Verification items for the finished model (mm, model axes). Face numbers are marked on the shaded views. Give positions to 0.01 mm unless a question says otherwise; leave off trailing zeros. Write each loop counter-clockwise with the first axis right and the second up, starting at its lowest first coordinate (ties: lowest second). Pieces come first, ordered by that corner, then holes. Notation, with made-up numbers: (-2.5, 57.25) -> (36.5, 57.25) arc R21 cw to (36.5, 74.25) -> close; hole circle Ø4 at (-23, 74). An arc over 180 degrees is marked (long way). Use one line per item in the form item = value. Start each with the question number.
(1) Scan lines: L1, parallel to Y at x = 0, z = 2; L2, parallel to X at y = -16, z = 2; L3, parallel to X at y = -8.5, z = 5.25. Record each from-to range of solid material in increasing order.
(2) Section check A-A, the plane z = 3. Record the cut outline in (x, y), plus the area to 3 significant figures.
(3) Section check B-B, the plane x = 8.5. Record the cut outline in (y, z), plus the area to 3 significant figures.
(4) Release check for a two-part mould opening along X. For the marked faces 1 and 2 record: pulls with the +X half, pulls with the -X half, needs draft (parallel to the pull), parting line crosses it, or undercut.
(5) Depth check by flat-ended pin: pin 1 Ø1 at (y, z) = (2.5, 4) entering from -X; pin 2 Ø8 at (x, y) = (24, 3) entering from +Z; pin 3 Ø20 at (x, y) = (0, 28.87) entering from +Z; pin 4 Ø1.5 at (x, z) = (-17.5, 5.5) entering from -Y. Enter the tip coordinate at first touch or a pass-through.
(6) Section check C-C, the plane y = 37.5. Record the cut outline in (x, z).
(7) Section check D-D, the plane x = -7. Record the cut outline in (y, z), plus the area to 3 significant figures.
from build123d import *

# Parameters (mm, degrees)
F0_R        = 11
F1_DEPTH    = 7
F2_T1_DEPTH = 7


# Not quite as in the source:
# - a fillet or chamfer that OpenCascade refuses, or shapes differently, is made with other operations: its cross-section is extruded or revolved along the edge and cut away or added


with BuildPart() as f1:
    # F0 (on Top) → F1 (new body)
    with BuildSketch(Plane.XY):
        with BuildLine():
            ThreePointArc((-17.5, -1.443375673), (-37.9903810568, -21.9337567297), (-10, -14.4337567297))
            Line((-10, -14.4337567297), (-14, -14.4337567297))
            ThreePointArc((-14, -14.4337567297), (-34.5262794416, -19.9337567297), (-19.5, -4.9074772881))
            Line((-19.5, -4.9074772881), (-17.5, -1.443375673))
        make_face()
        with BuildLine():
            ThreePointArc((-17.5, -1.443375673), (-12.0096189432, -6.9337567297), (-10, -14.4337567297))
            Line((-10, -14.4337567297), (10, -14.4337567297))
            ThreePointArc((10, -14.4337567297), (12.0096189432, -6.9337567297), (17.5, -1.443375673))
            Line((17.5, -1.443375673), (7.5, 15.8771324027))
            ThreePointArc((7.5, 15.8771324027), (0, 13.8675134595), (-7.5, 15.8771324027))
            Line((-7.5, 15.8771324027), (-17.5, -1.443375673))
        make_face()
        Circle(F0_R, mode=Mode.SUBTRACT)
        with BuildLine():
            Line((-14, -14.4337567297), (-10, -14.4337567297))
            ThreePointArc((-10, -14.4337567297), (-12.0096189432, -6.9337567297), (-17.5, -1.443375673))
            Line((-17.5, -1.443375673), (-19.5, -4.9074772881))
            ThreePointArc((-19.5, -4.9074772881), (-15.4737205584, -8.9337567297), (-14, -14.4337567297))
        make_face()
        with BuildLine():
            ThreePointArc((17.5, -1.443375673), (12.0096189432, -6.9337567297), (10, -14.4337567297))
            Line((10, -14.4337567297), (14, -14.4337567297))
            ThreePointArc((14, -14.4337567297), (15.4737205584, -8.9337567297), (19.5, -4.9074772881))
            Line((19.5, -4.9074772881), (17.5, -1.443375673))
        make_face()
        with BuildLine():
            Line((14, -14.4337567297), (10, -14.4337567297))
            ThreePointArc((10, -14.4337567297), (25, -29.4337567297), (40, -14.4337567297))
            ThreePointArc((40, -14.4337567297), (32.5, -1.443375673), (17.5, -1.443375673))
            Line((17.5, -1.443375673), (19.5, -4.9074772881))
            ThreePointArc((19.5, -4.9074772881), (30.5, -4.9074772881), (36, -14.4337567297))
            ThreePointArc((36, -14.4337567297), (25, -25.4337567297), (14, -14.4337567297))
        make_face()
        with BuildLine():
            ThreePointArc((15, 28.8675134595), (-7.5, 41.8578945162), (-7.5, 15.8771324027))
            Line((-7.5, 15.8771324027), (-5.5, 19.3412340179))
            ThreePointArc((-5.5, 19.3412340179), (-5.5, 38.3937929011), (11, 28.8675134595))
            ThreePointArc((11, 28.8675134595), (9.5262794416, 23.3675134595), (5.5, 19.3412340179))
            Line((5.5, 19.3412340179), (7.5, 15.8771324027))
            ThreePointArc((7.5, 15.8771324027), (12.9903810568, 21.3675134595), (15, 28.8675134595))
        make_face()
        with BuildLine():
            Line((-5.5, 19.3412340179), (-7.5, 15.8771324027))
            ThreePointArc((-7.5, 15.8771324027), (0, 13.8675134595), (7.5, 15.8771324027))
            Line((7.5, 15.8771324027), (5.5, 19.3412340179))
            ThreePointArc((5.5, 19.3412340179), (0, 17.8675134595), (-5.5, 19.3412340179))
        make_face()
    extrude(amount=F1_DEPTH)

    # F2: fillet of radius 15 on 6 edges, made by hand

    # F2_s2 → F2_t1 (join)
    with BuildSketch(Plane.XY):
        with BuildLine():
            ThreePointArc((12.9903810568, 6.3675134595), (10.9807621135, 13.8675134595), (12.9903810568, 21.3675134595))
            ThreePointArc((12.9903810568, 21.3675134595), (10.6066017178, 18.2609117417), (7.5, 15.8771324027))
            Line((7.5, 15.8771324027), (12.9903810568, 6.3675134595))
        make_face()
        with BuildLine():
            ThreePointArc((25, 0.5662432703), (17.5, 2.5758622135), (12.0096189432, 8.0662432703))
            Line((12.0096189432, 8.0662432703), (17.5, -1.443375673))
            ThreePointArc((17.5, -1.443375673), (21.1177143235, 0.0551306646), (25, 0.5662432703))
        make_face()
        with BuildLine():
            ThreePointArc((-12.9903810568, 21.3675134595), (-10.9807621135, 13.8675134595), (-12.9903810568, 6.3675134595))
            Line((-12.9903810568, 6.3675134595), (-7.5, 15.8771324027))
            ThreePointArc((-7.5, 15.8771324027), (-10.6066017178, 18.2609117417), (-12.9903810568, 21.3675134595))
        make_face()
        with BuildLine():
            ThreePointArc((-25, 0.5662432703), (-17.5, 2.5758622135), (-12.0096189432, 8.0662432703))
            Line((-12.0096189432, 8.0662432703), (-17.5, -1.443375673))
            ThreePointArc((-17.5, -1.443375673), (-21.1177143235, 0.0551306646), (-25, 0.5662432703))
        make_face()
        with BuildLine():
            ThreePointArc((-12.0096189432, -21.9337567297), (-6.5192378865, -16.443375673), (0.9807621135, -14.4337567297))
            Line((0.9807621135, -14.4337567297), (-10, -14.4337567297))
            ThreePointArc((-10, -14.4337567297), (-10.5111126057, -18.3160424063), (-12.0096189432, -21.9337567297))
        make_face()
        with BuildLine():
            ThreePointArc((-0.9807621135, -14.4337567297), (6.5192378865, -16.443375673), (12.0096189432, -21.9337567297))
            ThreePointArc((12.0096189432, -21.9337567297), (10.5111126057, -18.3160424063), (10, -14.4337567297))
            Line((10, -14.4337567297), (-0.9807621135, -14.4337567297))
        make_face()
    extrude(amount=F2_T1_DEPTH)


solid = f1.part
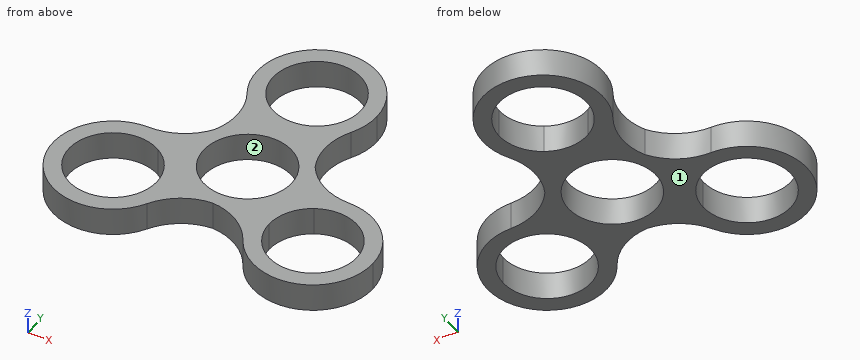
Completed:
q1.L1 = -14.47 to -11, 11 to 17.87, 39.87 to 43.87
q1.L2 = -39.92 to -35.89, -14.11 to -5.69, 5.69 to 14.11, 35.89 to 39.92
q1.L3 = -38.78 to -34.26, -15.74 to -6.98, 6.98 to 15.74, 34.26 to 38.78
q2.outline = (-25, 0.57) arc R15 ccw (long way) to (-12.01, -21.93) arc R15 cw to (0, -14.47) arc R15 cw to (12.01, -21.93) arc R15 ccw (long way) to (25, 0.57) arc R15 cw to (12.53, 7.23) arc R15 cw to (12.99, 21.37) arc R15 ccw (long way) to (-12.99, 21.37) arc R15 cw to (-12.53, 7.23) arc R15 cw to start; hole circle Ø22 at (-25, -14.43); hole circle Ø22 at (0, 0); hole circle Ø22 at (0, 28.87); hole circle Ø22 at (25, -14.43)
q2.area = 1,440 mm²
q3.outline = (-17.81, 0) -> (-6.98, 0) -> (-6.98, 7) -> (-17.81, 7) -> close; (6.98, 0) -> (21.89, 0) -> (21.89, 7) -> (6.98, 7) -> close; (35.85, 0) -> (41.23, 0) -> (41.23, 7) -> (35.85, 7) -> close
q3.area = 218 mm²
q4.face_1 = needs draft
q4.face_2 = undercut
q5.pin_1 = -18.6
q5.pin_2 = 7
q5.pin_3 = through
q5.pin_4 = -27.83
q6.outline = (-12.27, 0) -> (-6.82, 0) -> (-6.82, 7) -> (-12.27, 7) -> close; (6.82, 0) -> (12.27, 0) -> (12.27, 7) -> (6.82, 7) -> close
q7.outline = (-16.73, 0) -> (-8.49, 0) -> (-8.49, 7) -> (-16.73, 7) -> close; (8.49, 0) -> (20.38, 0) -> (20.38, 7) -> (8.49, 7) -> close; (37.35, 0) -> (42.13, 0) -> (42.13, 7) -> (37.35, 7) -> close
q7.area = 174 mm²
